Autodesk Inventor part; units mm, degrees
ref_plane "YZ Plane" through (0, 0, 0) normal (1, 0, 0) x (0, 1, 0)
ref_plane "XZ Plane" through (0, 0, 0) normal (0, 1, 0) x (-1, 0, 0)
ref_plane "XY Plane" through (0, 0, 0) normal (0, 0, 1) x (1, 0, 0)
sketch "Boceto1" plane through (0, 0, 0) normal (0, 1, 0) x (-1, 0, 0)
  line L0 (30, 55) -> (-30, 55)
  line L1 (-30, 55) -> (-30, -55)
  line L2 (-30, -55) -> (30, -55)
  line L3 (30, -55) -> (30, 55)
  line L4 (33, 58) -> (-33, 58)
  line L5 (-33, 58) -> (-33, -58)
  line L6 (-33, -58) -> (33, -58)
  line L7 (33, -58) -> (33, 58)
  point P0 (0, 0)
  point P1 (0, -55)
  point P2 (30, 0)
  dimension "d0" = 110
  dimension "d1" = 60
  dimension "d2" = 3
  dimension "d3" = 3
  dimension "d4" = 3
  dimension "d5" = 3
extrude "Extrusión1" add sketch "Boceto1" along normal blind 300
sketch "Boceto2" plane through (0, 300, 0) normal (0, 1, 0) x (1, 0, 0)
  line L0 (33, -58) -> (33, 58) construction
  line L1 (33, 58) -> (-33, 58) construction
  line L2 (-33, 58) -> (-33, -58) construction
  line L3 (-33, -58) -> (33, -58) construction
  line L4 (-30, -55) -> (-30, 55) construction
  line L5 (-30, 55) -> (30, 55) construction
  line L6 (30, 55) -> (30, -55) construction
  line L7 (30, -55) -> (-30, -55) construction
  line L8 (-30, -55) -> (-30, 55)
  line L9 (-30, 55) -> (30, 55)
  line L10 (30, 55) -> (30, 58)
  line L11 (30, 58) -> (-30, 58)
  line L12 (-30, 58) -> (-30, 55)
  point P0 (0, 0)
extrude "Extrusión2" cut sketch "Boceto2" against normal blind 295
extrude "Extrusión3" add sketch "Boceto1" along normal blind 5 contours L3 L2 L1 L0
sketch "Boceto4" plane through (30, 300, 55) normal (0, 0, -1) x (-1, 0, 0)
  line L0 (0, -295) -> (60, -295) construction
  line L1 (60, -295) -> (60, 0) construction
  line L2 (0, 0) -> (60, 0) construction
  line L3 (0, -295) -> (0, 0) construction
  line L4 (0, -295) -> (0, 0)
  line L5 (60, 0) -> (0, 0)
  line L6 (0, 0) -> (0, -5)
  line L7 (0, -5) -> (60, -5)
  line L8 (60, -5) -> (60, 0)
  point P0 (30, -300)
  dimension "d12" = 5
extrude "Extrusión4" add sketch "Boceto4" along normal blind 113
properties part number "caja"
Can you work these out from the model? Positions are in its coordinate system, mm. A direction names the side the tool comes from. Coordinates: 2 decimals unless noted, no trailing zeros. Loops run counter-clockwise (first coordinate to the right, second up) from the corner with the lowest first, then second, coordinate; pieces in that order, holes last. Notation, with made-up numbers: (-7, 84.5) -> (6, 84.5) arc R21 cw to (6, 102.5) -> close; hole circle Ø1 at (67.5, 59.25). An arc over 180 degrees is marked (long way). Answer as a JSON object with one key per item and string values.
1) Imagine slicing it at A-A (z = -21). Please give me the cut outline in (x, y).
Results:
{"outline": "(-33, 0) -> (33, 0) -> (33, 300) -> (-33, 300) -> close; hole (-30, 5) -> (30, 5) -> (30, 295) -> (-30, 295) -> close"}
2) For P1, Ø10, axis at x = -24, y = 39.5, coming from the -Z side, with a flat end and sliding along its axis, tell me the tip position at first contact or that it passes through.
Results:
{"P1": "stops at z = 55"}
3) If I drill on line 1 (X direction, y = 109, z = -51.5); line 2 (Y direction, x = -2, z = 32); line 3 (Z direction, x = 19, y = 76.5), over which ranges is the centre line in solid material (lowest first)?
Results:
{"line 1": "x = -33 to -30, 30 to 33", "line 2": "y = 0 to 5, 295 to 300", "line 3": "z = 55 to 58"}
4) Imagine slicing it at C-C (x = -15.5). Please give me the cut outline in (y, z).
Results:
{"outline": "(0, -58) -> (5, -58) -> (5, 55) -> (295, 55) -> (295, -58) -> (300, -58) -> (300, 58) -> (0, 58) -> close"}
5) Thinking about a two-plate mould opening in X: for faces 3 (the face through (0, 295, -1)), 4 (the face through (33, 148, 1)), 5 (the face through (0, 148, 58)), which applies, pulls with the +X half, pulls with the -X half, needs draft (parallel to the pull), parting line crosses it, or undercut?
Results:
{"face 3": "undercut", "face 4": "pulls with the +X half", "face 5": "needs draft"}
6) For faces 1 (the face through (0, 300, 1)), 2 (the face through (0, 5, -2)), which set-ups out of +Z, -Z, +X, -X, +Y, -Y let a thin tool reach every point of the face, with its end or its side?
Results:
{"face 1": "+Z, -Z, +X, -X, +Y", "face 2": "-Z"}
7) Imagine slicing it at B-B (y = 281). Please give me the cut outline in (x, z).
Results:
{"outline": "(-33, -58) -> (-30, -58) -> (-30, 55) -> (30, 55) -> (30, -58) -> (33, -58) -> (33, 58) -> (-33, 58) -> close"}
